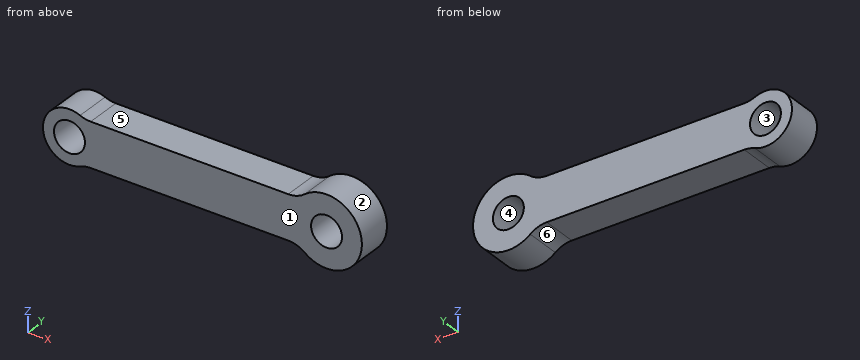
```python
from build123d import *

# Parameters (mm, degrees)
IZIM1_R                     = 1.75
Y_KSEKLIK_EKSTR_ZYON1_DEPTH = 4


with BuildPart() as part:
    # Çizim1 → Yükseklik-Ekstrüzyon1 (new body)
    with BuildSketch(Plane(origin=(0, 0, 0), x_dir=(1, 0, 0), z_dir=(0, 1, 0))):
        with BuildLine():
            Line((-10.218653411, -2.5), (4.071106479, -2.5))
            Line((4.071106479, -2.5), (11.17, -2.5))
            ThreePointArc((11.17, -2.5), (12.151980506, -2.665266452), (13.025768722, -3.142857143))
            ThreePointArc((13.025768722, -3.142857143), (19.500127019, 0), (13.025768722, 3.142857143))
            ThreePointArc((13.025768722, 3.142857143), (12.151980506, 2.665266452), (11.17, 2.5))
            Line((11.17, 2.5), (4.071106479, 2.5))
            Line((4.071106479, 2.5), (-10.218653411, 2.5))
            Line((-10.218653411, 2.5), (-11.17, 2.5))
            ThreePointArc((-11.17, 2.5), (-11.782372436, 2.563164969), (-12.368957881, 2.75))
            ThreePointArc((-12.368957881, 2.75), (-16.567915762, 0), (-12.368957881, -2.75))
            ThreePointArc((-12.368957881, -2.75), (-11.782372436, -2.563164969), (-11.17, -2.5))
            Line((-11.17, -2.5), (-10.218653411, -2.5))
        make_face()
        with Locations((-13.567915762, 0)):
            Circle(IZIM1_R, mode=Mode.SUBTRACT)
        with Locations((15.500127019, 0)):
            Circle(IZIM1_R, mode=Mode.SUBTRACT)
    extrude(amount=Y_KSEKLIK_EKSTR_ZYON1_DEPTH)


solid = part.part
```
Geometry: final body of the model. Coordinates: model frame, mm. Face numbers are marked on the shaded views. A direction names the side the tool comes from. Give positions to 0.01 mm unless a question says otherwise; leave off trailing zeros. Order: outer loops, then holes, each group sorted by start corner. A loop starts at its lowest first (then second) coordinate and runs counter-clockwise, first axis right, second up. Notation, with made-up numbers: (23.5, 75.5) -> (30.5, 75.5) arc R16 cw to (30.5, 85.5) -> close; hole circle Ø4 at (24, 25.5). An arc over 180 degrees is marked (long way). Write each question's results on one line, items separated by ' | '. Start each with the question number.
1) First-contact query: pin 1 (4 mm diameter, centred on x = -4, z = -3, fed in from -Y); pin 2 (3 mm diameter, centred on x = 15.5, z = 0, fed in from +Y); pin 3 (1.2 mm diameter, centred on x = 2.5, y = 3, fed in from -Z). Flat tips, straight axial feed; report the tip coordinate or a pass-through.
2) Section A-A (z = 0). Return loops of the section in (x, y), then the cut area to 3 significant figures.
3) Line query: line 1 (X direction, y = 2.35, z = 0); line 2 (X direction, y = 3.65, z = 0.75); line 3 (Z direction, x = 17, y = 1.95). Output: solid intervals per line, ascending. Write a range as from..to.
4) Section B-B (y = 1.35). Return loops of the section in (x, z).
5) Draft query along X for the marked faces 1, 2 and 3. Return one class per face: pulls with the +X half, pulls with the -X half, needs draft (parallel to the pull), parting line crosses it, or undercut.
6) Set-up query: the marked faces 4, 5 and 6. Return all of +Z, -Z, +X, -X, +Y, -Y with unobstructed straight access to the full face (end or side cutting, diameter ignored); none if empty.
7) Section C-C (x = 4). Return loops of the section in (y, z).
Calculated:
1) pin 1: y = 0 | pin 2: through | pin 3: z = -2.5
2) outline: (-16.57, 0) -> (-15.32, 0) -> (-15.32, 4) -> (-16.57, 4) -> close; (-11.82, 0) -> (13.75, 0) -> (13.75, 4) -> (-11.82, 4) -> close; (17.25, 0) -> (19.5, 0) -> (19.5, 4) -> (17.25, 4) -> close | area: 116 mm2
3) line 1: -16.57..-15.32, -11.82..13.75, 17.25..19.5 | line 2: -16.47..-15.15, -11.99..13.92, 17.08..19.43 | line 3: -3.71..-0.9, 0.9..3.71
4) outline: (-12.37, -2.75) arc R3 cw to (-11.17, -2.5) -> (11.17, -2.5) arc R3 cw to (13.03, -3.14) arc R4 ccw (long way) to (13.03, 3.14) arc R3 cw to (11.17, 2.5) -> (-11.17, 2.5) arc R3 cw to (-12.37, 2.75) arc R3 ccw (long way) to start; hole circle Ø3.5 at (-13.57, 0); hole circle Ø3.5 at (15.5, 0)
5) face 1: needs draft | face 2: parting line crosses it | face 3: undercut
6) face 4: +Y, -Y | face 5: +Z, +Y, -Y | face 6: -Z, +Y, -Y
7) outline: (0, -2.5) -> (4, -2.5) -> (4, 2.5) -> (0, 2.5) -> close
